from build123d import *

# Parameters (mm, degrees)
SKETCH1_R           = 75
SKETCH1_R_2         = 15
BOSS_EXTRUDE1_DEPTH = 30
CUT_EXTRUDE1_DEPTH  = 30


with BuildPart() as part:
    # Sketch1 → Boss-Extrude1 (new body)
    with BuildSketch(Plane.XY):
        Circle(SKETCH1_R)
        Circle(SKETCH1_R_2, mode=Mode.SUBTRACT)
    extrude(amount=BOSS_EXTRUDE1_DEPTH)

    # Sketch3 → Cut-Extrude1 (cut)
    with BuildSketch(Plane.XY.offset(30)):
        with BuildLine():
            ThreePointArc((20, 0), (41.783391285, -1.00391685), (61.214489176, -10.901210401))
            ThreePointArc((61.214489176, -10.901210401), (66.308819549, 1.397591077), (61.214489176, 13.696392555))
            ThreePointArc((61.214489176, 13.696392555), (38.925210815, 11.909686918), (20, 0))
        make_face()
        with BuildLine():
            ThreePointArc((0, 20), (11.265284699, 40.943063639), (13.975910771, 64.568707761))
            ThreePointArc((13.975910771, 64.568707761), (1.257831969, 69.836708488), (-11.460246832, 64.568707761))
            ThreePointArc((-11.460246832, 64.568707761), (-3.286702106, 42.912646975), (0, 20))
        make_face()
        with BuildLine():
            ThreePointArc((-20, 0), (-40.056959125, -10.422925538), (-62.612080253, -8.944582893))
            ThreePointArc((-62.612080253, -8.944582893), (-68.838529986, 1.739113534), (-65.686780623, 13.696392555))
            ThreePointArc((-65.686780623, 13.696392555), (-44.364425117, 1.774511129), (-20, 0))
        make_face()
        with BuildLine():
            ThreePointArc((0, -20), (10.122111276, -40.697980205), (9.503619324, -63.730153115))
            ThreePointArc((9.503619324, -63.730153115), (-2.795182154, -68.824483488), (-15.093983632, -63.730153115))
            ThreePointArc((-15.093983632, -63.730153115), (-5.375443737, -42.614612263), (0, -20))
        make_face()
    extrude(amount=-CUT_EXTRUDE1_DEPTH, mode=Mode.SUBTRACT)


solid = part.part
Geometry check sheet. Reference: the model listing, model coordinates, mm. A direction names the side the tool comes from. Coordinates: 2 decimals unless noted, no trailing zeros. Order: outer loops, then holes, each group sorted by start corner. A loop starts at its lowest first (then second) coordinate and runs counter-clockwise, first axis right, second up. Notation, with made-up numbers: (-22, 0) -> (18, 0) arc R15 cw to (18, 19) -> close; hole circle Ø9 at (62.5, -12). An arc over 180 degrees is marked (long way). Use a Markdown table: item, result. Add a question column.
1. Set-up check for faces 4 (the face through (66.308, 1.206, 15.21)), 5 (the face through (-1, -16, 0)): record each of +Z, -Z, +X, -X, +Y, -Y from which the full face is reachable in a straight line by a thin tool's end or side.
2. Cross-section at B-B (x = 28). Enter the section's corners in (y, z).
3. Cross-section at C-C (y = -53.5). Enter the section's corners in (x, z).
4. Material ranges on L1, parallel to X at y = -7.5, z = 27; L2, parallel to X at y = -40, z = 5.5 (3 decimals); L3, parallel to X at y = 61, z = 10.75, recorded low to high.
5. Mould release check, pull along Y, two halves, no side actions. Record for faces 1 (the face through (-1, -16, 30)), 2 (the face through (11.164, 40.624, 15.21)), 3 (the face through (-9.764, 74.362, 14.79)): pulls with the +Y half, pulls with the -Y half, needs draft (parallel to the pull), parting line crosses it, or undercut.
6. Cross-section at A-A (z = 3.5). Enter the section's corners in (x, y), and give its area (3 significant figures).
7. Go/stop test with flat-tipped pins: pin 1 Ø2 at (x, z) = (34, 12.5) entering from +Y; pin 2 Ø3 at (x, z) = (10.5, 25.5) entering from -Y; pin 3 Ø1 at (x, z) = (-4.5, 16) entering from +Y. Record where each tip stops, or that it passes through.
Filled sheet:
| question | item | result |
|---|---|---|
| 1 | face 4 | +Z, -Z |
| 1 | face 5 | -Z, +X, -X, +Y, -Y |
| 2 | outline | (-69.58, 0) -> (0.71, 0) -> (0.71, 30) -> (-69.58, 30) -> close; (6.62, 0) -> (69.58, 0) -> (69.58, 30) -> (6.62, 30) -> close |
| 3 | outline | (-52.56, 0) -> (-9.75, 0) -> (-9.75, 30) -> (-52.56, 30) -> close; (11.16, 0) -> (52.56, 0) -> (52.56, 30) -> (11.16, 30) -> close |
| 4 | L1 | -74.62 to -64.26, -31.19 to -12.99, 12.99 to 56.53, 63.86 to 74.62 |
| 4 | L2 | -63.443 to -4.507, 9.965 to 63.443 |
| 4 | L3 | -43.63 to -9.73, 14.14 to 43.63 |
| 5 | face 1 | needs draft |
| 5 | face 2 | undercut |
| 5 | face 3 | parting line crosses it |
| 6 | outline | circle Ø150 at (0, 0); hole (-65.69, 13.7) arc R16.16 ccw to (-62.61, -8.94) arc R42.01 ccw to (-20, 0) arc R56.33 cw to start; hole (-15.09, -63.73) arc R17.39 ccw to (9.5, -63.73) arc R48.3 ccw to (0, -20) arc R117.6 cw to start; hole circle Ø30 at (0, 0); hole (-11.46, 64.57) arc R106.19 cw to (0, 20) arc R63.08 ccw to (13.98, 64.57) arc R17.99 ccw to start; hole (20, 0) arc R51.69 cw to (61.21, -10.9) arc R17.39 ccw to (61.21, 13.7) arc R46.87 ccw to start |
| 6 | area | 14,300 mm2 |
| 7 | pin 1 | y = 67.35 |
| 7 | pin 2 | y = -74.46 |
| 7 | pin 3 | y = 74.89 |
